Check sheet for the modelled part. Datum: model origin and axes. Units: mm. Round coordinates to 2 decimals unless told otherwise and drop trailing zeros. Write each loop counter-clockwise with the first axis right and the second up, starting at its lowest first coordinate (ties: lowest second). Pieces come first, ordered by that corner, then holes.
Item 1: Material ranges on line 1 (Y direction, x = -0.75, z = 2.35) (3 decimals); line 2 (Z direction, x = -1.4, y = 1.4); line 3 (Z direction, x = -1.25, y = 1.75), recorded low to high.
Item 2: Release check for a two-part mould opening along X. For faces 1 (the flat face through (0, 3, 2.55)), 2 (the flat face through (0, 3.45, 0)), 3 (the flat face through (-2.25, 2.24, -1.11)) record: +X half, -X half, draft (parallel to the pull), parting line (faces both ways), or undercut.
Item 3: Cross-section at A-A on z = -15. Enter the section's corners in (x, y).
Item 4: Go/stop test with flat-tipped pins: pin 1 Ø0.5 at (x, z) = (-0.5, 2.5) entering from -Y; pin 2 Ø0.5 at (x, y) = (2, 1) entering from +Z; pin 3 Ø0.9 at (x, y) = (1, 3.5) entering from -Z. Record where each tip stops, or that it passes through.
from build123d import *

# Parameters (mm, degrees)
SKETCH1_W                        = 4.5
SKETCH1_H                        = 3.05
BOSS_EXTRUDE1_DEPTH              = 0.6
SKETCH2_W                        = 0.94
SKETCH2_H                        = 1.55
BOSS_EXTRUDE2_DEPTH              = 0.3
SKETCH3_W                        = 0.94
SKETCH3_H                        = 1.55
BOSS_EXTRUDE3_DEPTH              = 0.3
SKETCH4_W                        = 2.62
SKETCH4_H                        = 1.55
CUT_EXTRUDE1_DEPTH               = 0.3
SKETCH5_W                        = 3.4
SKETCH5_H                        = 2.68
BOSS_EXTRUDE4_DEPTH              = 3.9
SKETCH6_W                        = 2.2
SKETCH6_H                        = 0.8
BOSS_EXTRUDE5_DEPTH              = 0.55
SKETCH7_W                        = 2.2
SKETCH7_H                        = 0.8
BOSS_EXTRUDE6_DEPTH              = 0.55
SKETCH8_W                        = 0.3
SKETCH8_H                        = 1.35
CUT_EXTRUDE2_DEPTH               = 6.968877616
CUT_EXTRUDE3_DEPTH               = 6.968877616
SKETCH10_W                       = 0.5
SKETCH10_H                       = 0.59
BOSS_EXTRUDE7_DEPTH              = 0.14
SKETCH11_W                       = 1.2
SKETCH11_H                       = 0.6
BOSS_EXTRUDE8_DEPTH              = 0.35
SKETCH12_W                       = 0.5
SKETCH12_H                       = 0.59
BOSS_EXTRUDE9_DEPTH              = 0.14
DRAFT1_ANGLE                     = 45
F_0_55_0_55_DIAMETER_HOLE1_D     = 0.55
F_0_55_0_55_DIAMETER_HOLE1_DEPTH = 0.4
RIB1_START                       = -0.19
RIB1_OUTLINE_W                   = 1.55
RIB1_OUTLINE_H                   = 0.6
RIB1_DEPTH                       = 0.38
SKETCH16_R                       = 0.5
BOSS_EXTRUDE10_DEPTH             = 80
SKETCH17_W                       = 0.960697218
SKETCH17_H                       = 0.952555717
CUT_EXTRUDE4_DEPTH               = 0.37


# Read off the part's stored shape, not the designer's step: Rib1
with BuildPart() as part:
    # Sketch1 → Boss-Extrude1 (new body)
    with BuildSketch(Plane(origin=(0, 0, -1.65), x_dir=(-1, 0, 0), z_dir=(0, 0, -1))):
        with Locations((0, 1.925)):
            Rectangle(SKETCH1_W, SKETCH1_H)
    extrude(amount=-BOSS_EXTRUDE1_DEPTH)

    # Sketch2 → Boss-Extrude2 (add)
    with BuildSketch(Plane(origin=(0, 0, -1.65), x_dir=(-1, 0, 0), z_dir=(0, 0, -1))):
        with Locations((1.78, 2.225)):
            Rectangle(SKETCH2_W, SKETCH2_H)
    extrude(amount=BOSS_EXTRUDE2_DEPTH)

    # Sketch3 → Boss-Extrude3 (add)
    with BuildSketch(Plane(origin=(0, 0, -1.65), x_dir=(-1, 0, 0), z_dir=(0, 0, -1))):
        with Locations((-1.78, 2.225)):
            Rectangle(SKETCH3_W, SKETCH3_H)
    extrude(amount=BOSS_EXTRUDE3_DEPTH)

    # Sketch4 → Cut-Extrude1 (cut)
    with BuildSketch(Plane(origin=(0, 0, -1.65), x_dir=(-1, 0, 0), z_dir=(0, 0, -1))):
        with Locations((0, 2.225)):
            Rectangle(SKETCH4_W, SKETCH4_H)
    extrude(amount=-CUT_EXTRUDE1_DEPTH, mode=Mode.SUBTRACT)

    # Sketch5 → Boss-Extrude4 (add)
    with BuildSketch(Plane.XY.offset(-1.05)):
        with Locations((0, 2.11)):
            Rectangle(SKETCH5_W, SKETCH5_H)
    extrude(amount=BOSS_EXTRUDE4_DEPTH)

    # Sketch6 → Boss-Extrude5 (add)
    with BuildSketch(Plane(origin=(1.7, 0, 0), x_dir=(0, 0, -1), z_dir=(1, 0, 0))):
        with Locations((-0.05, 2.5)):
            Rectangle(SKETCH6_W, SKETCH6_H)
    extrude(amount=BOSS_EXTRUDE5_DEPTH)

    # Sketch7 → Boss-Extrude6 (add)
    with BuildSketch(Plane.ZY.offset(1.7)):
        with Locations((0.05, 2.5)):
            Rectangle(SKETCH7_W, SKETCH7_H)
    extrude(amount=BOSS_EXTRUDE6_DEPTH)

    # Sketch8 → Cut-Extrude2 (cut, through all)
    with BuildSketch(Plane.ZY.offset(1.7)):
        with Locations((2.7, 2.775)):
            Rectangle(SKETCH8_W, SKETCH8_H)
    extrude(amount=-CUT_EXTRUDE2_DEPTH, mode=Mode.SUBTRACT)

    # Sketch9 → Cut-Extrude3 (cut, through all)
    with BuildSketch(Plane.ZY.offset(1.7)):
        Polygon((1.4411, 0.77), (1.919971259, 0.77), (1.919971259, 1.45), (1.469971259, 1.45), (1.469971259, 1.1), align=None)
    extrude(amount=-CUT_EXTRUDE3_DEPTH, mode=Mode.SUBTRACT)

    # Sketch10 → Boss-Extrude7 (add)
    with BuildSketch(Plane(origin=(0, 3.45, 0), x_dir=(-1, 0, 0), z_dir=(0, 1, 0))):
        with Locations((1.45, 1.595)):
            Rectangle(SKETCH10_W, SKETCH10_H)
    extrude(amount=BOSS_EXTRUDE7_DEPTH)

    # Sketch11 → Boss-Extrude8 (add)
    with BuildSketch(Plane(origin=(0, 3.45, 0), x_dir=(-1, 0, 0), z_dir=(0, 1, 0))):
        with Locations((0, -1.35)):
            Rectangle(SKETCH11_W, SKETCH11_H)
    extrude(amount=BOSS_EXTRUDE8_DEPTH)

    # Sketch12 → Boss-Extrude9 (add)
    with BuildSketch(Plane(origin=(0, 3.45, 0), x_dir=(-1, 0, 0), z_dir=(0, 1, 0))):
        with Locations((-1.45, 1.595)):
            Rectangle(SKETCH12_W, SKETCH12_H)
    extrude(amount=BOSS_EXTRUDE9_DEPTH)

    # Draft1
    draft1_faces = [part.faces().sort_by_distance(p)[0] for p in [
        (0, 2.1, 2.7),
    ]]
    draft(draft1_faces, Plane(origin=(2.250025, 3.45, 2.55), x_dir=(0, 1, 0), z_dir=(0, 0, 1)), DRAFT1_ANGLE)

    # Ø0.55 (0.55) Diameter Hole1
    with Locations(Plane.XY.offset(2.55)):
        with Locations((-0.75, 2.55), (0.75, 2.55)):
            Hole(F_0_55_0_55_DIAMETER_HOLE1_D / 2, depth=F_0_55_0_55_DIAMETER_HOLE1_DEPTH)

    # Rib1 outline → Rib1 (add)
    with BuildSketch(Plane(origin=(0, 0, 0), x_dir=(0, -1, 0), z_dir=(-1, 0, 0)).offset(RIB1_START)):
        with Locations((-2.225, -1.65)):
            Rectangle(RIB1_OUTLINE_W, RIB1_OUTLINE_H)
    extrude(amount=RIB1_DEPTH)

    # Sketch16 → Boss-Extrude10 (add)
    with BuildSketch(Plane(origin=(0, 0, -1.35), x_dir=(-1, 0, 0), z_dir=(0, 0, -1))):
        with Locations(Location((-0.75, 2.216914792, 0), (0, 0, 90))):
            Circle(SKETCH16_R)
        with Locations(Location((0.75, 2.216914792, 0), (0, 0, 90))):
            Circle(SKETCH16_R)
    extrude(amount=BOSS_EXTRUDE10_DEPTH)

    # Sketch17 → Cut-Extrude4 (cut)
    with BuildSketch(Plane.XZ.offset(-0.4)):
        with Locations((0.713949263, -1.321573248)):
            Rectangle(SKETCH17_W, SKETCH17_H)
    extrude(amount=-CUT_EXTRUDE4_DEPTH, mode=Mode.SUBTRACT)


solid = part.part
Response values:
1. line 1: y = 0.77 to 2.275, 2.825 to 3.45
1. line 2: z = -1.65 to 1.47, 1.92 to 2.85
1. line 3: z = -1.35 to 2.85
2. face 1: draft
2. face 2: undercut
2. face 3: -X half
3. outline: circle Ø1 at (-0.75, 2.22); circle Ø1 at (0.75, 2.22)
4. pin 1: stops at y = 0.77
4. pin 2: stops at z = -1.05
4. pin 3: stops at z = -1.65
